Verification items for the finished model (mm, model axes). Face numbers are marked on the shaded views. Give positions to 0.01 mm unless a question says otherwise; leave off trailing zeros. Write each loop counter-clockwise with the first axis right and the second up, starting at its lowest first coordinate (ties: lowest second). Pieces come first, ordered by that corner, then holes. Notation, with made-up numbers: (40.5, 81) -> (48.5, 81) arc R10 cw to (48.5, 99) -> close; hole circle Ø10 at (49, 65.25). An arc over 180 degrees is marked (long way). Answer as CSV lines item,"result".
Autodesk Inventor part; units mm, degrees
ref_plane "YZ Plane" through (0, 0, 0) normal (1, 0, 0) x (0, 1, 0)
ref_plane "XZ Plane" through (0, 0, 0) normal (0, 1, 0) x (-1, 0, 0)
ref_plane "XY Plane" through (0, 0, 0) normal (0, 0, 1) x (1, 0, 0)
sketch "Sketch1" plane through (0, 0, 0) normal (0, 1, 0) x (-1, 0, 0)
  circle A0 centre (0, 0) radius 16.5 construction
  circle A1 centre (0, 0) radius 3.3
  arc A2 (-0.8286, 18.2098) -> (0.8286, 18.2098) centre (0, 16.5) ccw
  line L0 (0, 0) -> (9.875, 17.104) construction
  line L1 (0, 0) -> (-9.875, 17.104) construction
  line L2 (0, 0) -> (-17.104, 9.875) construction
  line L3 (0, 0) -> (17.104, 9.875) construction
  line L4 (-19.75, 0) -> (19.75, 0) construction
  circle A3 centre (0, -16.5) radius 1.75
  circle A4 centre (14.2894, 8.25) radius 1.75
  circle A5 centre (-14.2894, 8.25) radius 1.75
  arc A6 (8.3873, 16.1844) -> (9.8225, 15.3559) centre (8.25, 14.2894) ccw
  arc A7 (-9.8225, 15.3559) -> (-8.3873, 16.1844) centre (-8.25, 14.2894) ccw
  line L5 (0, 0) -> (0.75, 16.4829) construction
  line L6 (-0.75, 16.4829) -> (0, 0) construction
  line L7 (-7.592, 14.6496) -> (0, 0) construction
  line L8 (-8.891, 13.8996) -> (0, 0) construction
  line L9 (7.592, 14.6496) -> (0, 0) construction
  line L10 (8.891, 13.8996) -> (0, 0) construction
  line L11 (-8.3873, 16.1844) -> (-9.0873, 17.5352)
  line L12 (-9.8225, 15.3559) -> (-10.6422, 16.6375)
  line L13 (-0.8286, 18.2098) -> (-0.8977, 19.7296)
  line L14 (0.8286, 18.2098) -> (0.8977, 19.7296)
  line L15 (8.3873, 16.1844) -> (9.0873, 17.5352)
  line L16 (9.8225, 15.3559) -> (10.6422, 16.6375)
  arc A8 (9.0873, 17.5352) -> (0.8977, 19.7296) centre (0, 0) ccw
  arc A9 (-0.8977, 19.7296) -> (-9.0873, 17.5352) centre (0, 0) ccw
  arc A10 (-10.6422, 16.6375) -> (10.6422, 16.6375) centre (0, 0) ccw
  dimension "d1" = 33
  dimension "d2" = 6.6
  dimension "d3" = 3.8
  dimension "d4" = 30
  dimension "d5" = 60
  dimension "d6" = 60
  dimension "d7" = 30
  dimension "d8" = 3.5
  dimension "d9" = 3.5
  dimension "d10" = 3.5
  dimension "d11" = 3.8
  dimension "d12" = 3.8
  dimension "d13" = 0.75
  dimension "d14" = 0.75
  dimension "d15" = 0.75
  dimension "d16" = 0.75
  dimension "d17" = 0.75
  dimension "d18" = 0.75
  dimension "d20" = 19.75
  dimension "d21" = 19.75
  dimension "d22" = 19.75
extrude "Extrusion1" add sketch "Sketch1" along normal blind 6.35
fillet "Fillet1" radius 0.9 6 edges at (9.0873, 3.175, 17.5352) (10.6422, 3.175, 16.6375) (-0.8977, 3.175, 19.7296) (0.8977, 3.175, 19.7296) (-10.6422, 3.175, 16.6375) (-9.0873, 3.175, 17.5352)
fillet "Fillet2" radius 0.9 6 edges at (-9.8225, 3.175, 15.3559) (-0.8286, 3.175, 18.2098) (-8.3873, 3.175, 16.1844) (0.8286, 3.175, 18.2098) (8.3873, 3.175, 16.1844) (9.8225, 3.175, 15.3559)
properties part number "UpperPlate"
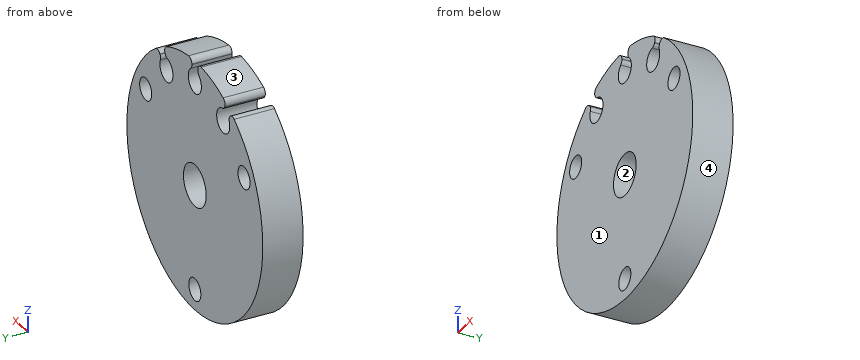
1) Section check D-D (x = 7.5). Record the boundary of the cut face in (y, z), and give its area (3 significant figures).
Reported:
outline,"(0, -18.27) -> (6.35, -18.27) -> (6.35, 12.54) -> (0, 12.54) -> close; (0, 16.04) -> (6.35, 16.04) -> (6.35, 18.27) -> (0, 18.27) -> close"
area,"210 mm²"
2) Section check A-A (x = 0). Record the boundary of the cut face in (y, z).
Reported:
outline,"(0, -19.75) -> (6.35, -19.75) -> (6.35, -18.25) -> (0, -18.25) -> close; (0, -14.75) -> (6.35, -14.75) -> (6.35, -3.3) -> (0, -3.3) -> close; (0, 3.3) -> (6.35, 3.3) -> (6.35, 14.6) -> (0, 14.6) -> close"
3) Section check C-C (y = 2.75). Record the boundary of the cut face in (x, z), and give its area (3 significant figures).
Reported:
outline,"(-11.42, 16.11) arc R19.75 ccw (long way) to (11.42, 16.11) arc R0.9 ccw to (10.15, 15.86) -> (10.1, 15.79) arc R0.9 ccw to (10.02, 14.98) arc R1.9 cw (long way) to (7.96, 16.17) arc R0.9 ccw to (8.62, 16.64) -> (8.66, 16.72) arc R0.9 ccw to (8.24, 17.95) arc R19.75 ccw to (1.84, 19.66) arc R0.9 ccw to (0.86, 18.81) -> (0.85, 18.73) arc R0.9 ccw to (1.19, 17.98) arc R1.9 cw (long way) to (-1.19, 17.98) arc R0.9 ccw to (-0.85, 18.73) -> (-0.86, 18.81) arc R0.9 ccw to (-1.84, 19.66) arc R19.75 ccw to (-8.24, 17.95) arc R0.9 ccw to (-8.66, 16.72) -> (-8.62, 16.64) arc R0.9 ccw to (-7.96, 16.17) arc R1.9 cw (long way) to (-10.02, 14.98) arc R0.9 ccw to (-10.1, 15.79) -> (-10.15, 15.86) arc R0.9 ccw to start; hole circle Ø3.5 at (-14.29, 8.25); hole circle Ø6.6 at (0, 0); hole circle Ø3.5 at (0, -16.5); hole circle Ø3.5 at (14.29, 8.25)"
area,"1,120 mm²"
4) Section check B-B (z = 0). Record the boundary of the cut face in (x, y).
Reported:
outline,"(-19.75, 0) -> (-3.3, 0) -> (-3.3, 6.35) -> (-19.75, 6.35) -> close; (3.3, 0) -> (19.75, 0) -> (19.75, 6.35) -> (3.3, 6.35) -> close"
5) Draft check along X on the marked faces 1, 2, 3 and 4. Enter one of: +X half, -X half, draft (parallel to the pull), parting line (faces both ways), or undercut.
Reported:
face 1,"draft"
face 2,"undercut"
face 3,"-X half"
face 4,"parting line"
6) Scan lines: line 1 along Z through (x, y) = (0, 3.5); line 2 along X through (y, z) = (3, 9); line 3 along X through (y, z) = (5, 16). Record each from-to range of solid material in increasing order.
Reported:
line 1,"-19.75 to -18.25, -14.75 to -3.3, 3.3 to 14.6"
line 2,"-17.58 to -15.87, -12.71 to 12.71, 15.87 to 17.58"
line 3,"-11.58 to -10.26, -7.42 to -1.83, 1.83 to 7.42, 10.26 to 11.58"
7) Depth check by flat-ended pin: pin 1 (6 mm diameter, centred on x = 5, z = 8, fed in from -Y); pin 2 (2 mm diameter, centred on x = 14.29, z = 8.25, fed in from +Y); pin 3 (3 mm diameter, centred on y = 4, z = -8.5, fed in from -X); pin 4 (3 mm diameter, centred on x = 6.5, y = 5, fed in from +Z). Enter the tip coordinate at first touch or a pass-through.
Reported:
pin 1,"y = 0"
pin 2,"through"
pin 3,"x = -18.47"
pin 4,"z = 19.11"
